Autodesk Inventor part; units mm, degrees
ref_plane "YZ Plane" through (0, 0, 0) normal (1, 0, 0) x (0, 1, 0)
ref_plane "XZ Plane" through (0, 0, 0) normal (0, 1, 0) x (-1, 0, 0)
ref_plane "XY Plane" through (0, 0, 0) normal (0, 0, 1) x (1, 0, 0)
sketch "Sketch1" plane through (0, 0, 0) normal (0, 1, 0) x (-1, 0, 0)
  line L0 (0, 0) -> (9, 0)
  line L1 (9, 0) -> (9, -30)
  line L2 (9, -30) -> (0, -30)
  line L3 (0, -30) -> (0, 0)
  dimension "d0" = 9
  dimension "d1" = 30
extrude "Extrusion1" add sketch "Sketch1" along normal blind 9
sketch "Sketch2" plane through (0, 0, 0) normal (0, -1, 0) x (1, 0, 0)
  line L0 (-3, -3) -> (-6, -3)
  line L1 (-6, -3) -> (-6, -27)
  line L2 (-6, -27) -> (-3, -27)
  line L3 (-3, -27) -> (-3, -3)
  line L4 (0, 0) -> (0, -30)
  line L5 (-9, -30) -> (-9, 0)
  line L6 (-9, 0) -> (0, 0)
  line L7 (0, -30) -> (-9, -30)
  point P0 (-4.5, 0)
  point P1 (-4.5, -30)
  dimension "d4" = 3
  dimension "d5" = 3
  dimension "d6" = 3
  dimension "d7" = 3
extrude "Extrusion2" cut sketch "Sketch2" against normal blind 1 contours L3 L2 L1 L0
fillet "Fillet1" radius 1 4 edges at (-6, 0.5, -27) (-3, 0.5, -27) (-6, 0.5, -3) (-3, 0.5, -3)
sketch "Sketch3" plane through (0, 9, 0) normal (0, 1, 0) x (1, 0, 0)
  line L0 (-5, 3) -> (-4, 3)
  line L1 (-3, 4) -> (-3, 26)
  line L2 (-4, 27) -> (-5, 27)
  line L3 (-6, 26) -> (-6, 4)
  arc A0 (-6, 4) -> (-5, 3) centre (-5, 4) ccw
  arc A1 (-5, 27) -> (-6, 26) centre (-5, 26) ccw
  arc A2 (-3, 26) -> (-4, 27) centre (-4, 26) ccw
  arc A3 (-4, 3) -> (-3, 4) centre (-4, 4) ccw
  line L4 (0, 0) -> (0, 30)
  line L5 (-9, 30) -> (-9, 0)
  line L6 (-9, 0) -> (0, 0)
  line L7 (0, 30) -> (-9, 30)
  point P0 (-4.5, 0)
  point P1 (-4.5, 3)
  point P2 (-4.5, 30)
  point P3 (-4.5, 27)
  dimension "d11" = 1
  dimension "d12" = 1
  dimension "d13" = 3
  dimension "d14" = 3
  dimension "d15" = 3
  dimension "d16" = 3
extrude "Extrusion3" cut sketch "Sketch3" against normal blind 1 contours A0 L3 A1 L2 A2 L1 A3 L0
properties part number "oled_support"
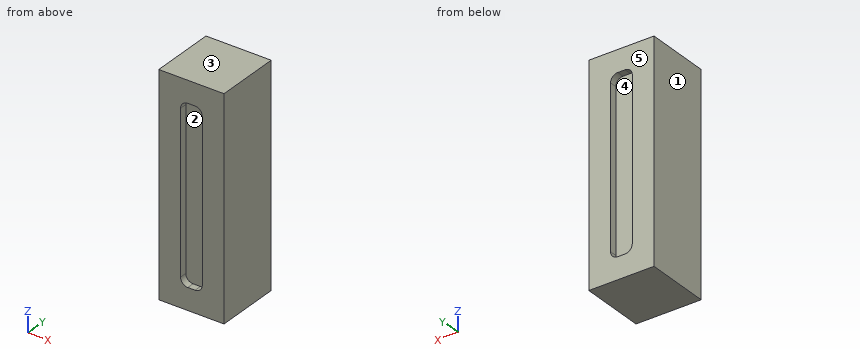
Geometry: final body of the model. Coordinates: model frame, mm. Face numbers are marked on the shaded views. A direction names the side the tool comes from. Coordinates: 2 decimals unless noted, no trailing zeros. Loops run counter-clockwise (first coordinate to the right, second up) from the corner with the lowest first, then second, coordinate; pieces in that order, holes last. Notation, with made-up numbers: (-25, 86) -> (5, 86) arc R9 cw to (5, 98) -> close; hole circle Ø10 at (82, 16.5). An arc over 180 degrees is marked (long way). Use a Markdown table: item, result. Add a question column.
(1) Pin query (flat end, axial travel): pin 1 Ø2.5 at (x, z) = (-4.5, -10) entering from +Y. Return the tip coordinate at first contact, or that it passes through.
(2) Line query: line 1 along X through (y, z) = (0.75, -25.75); line 2 along Y through (x, z) = (-5.5, -17); line 3 along Z through (x, y) = (-3.75, 8.75). Output: solid intervals per line, ascending.
(3) Section query A-A, the plane z = -18.25. Return loops of the section in (x, y), plus the area to 3 significant figures.
(4) Access query for the marked faces 4 and 5. Directions: +Z, -Z, +X, -X, +Y, -Y. A direction counts if a zero-diameter tool reaches every point of the face in a straight line with its end or side. Return the directions, or none.
(5) Mould query, pull axis X, two halves, no side actions, for the marked faces 1, 2 and 3. Classes: pulls with the +X half, pulls with the -X half, needs draft (parallel to the pull), parting line crosses it, or undercut.
Answer:
| question | item | result |
|---|---|---|
| 1 | pin 1 | stops at y = 8 |
| 2 | line 1 | x = -9 to -6, -3 to 0 |
| 2 | line 2 | y = 1 to 8 |
| 2 | line 3 | z = -30 to -26.97, -3.03 to 0 |
| 3 | outline | (-9, 0) -> (-6, 0) -> (-6, 1) -> (-3, 1) -> (-3, 0) -> (0, 0) -> (0, 9) -> (-3, 9) -> (-3, 8) -> (-6, 8) -> (-6, 9) -> (-9, 9) -> close |
| 3 | area | 75.0 mm^2 |
| 4 | face 4 | +Y |
| 4 | face 5 | +Z, -Z, +X, -X, +Y |
| 5 | face 1 | pulls with the -X half |
| 5 | face 2 | undercut |
| 5 | face 3 | needs draft |
